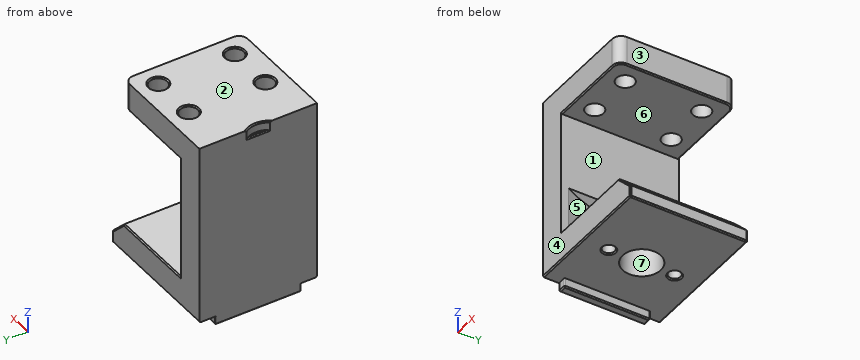
from build123d import *

# Parameters (mm, degrees)
SKETCH_1_R          = 3.2375
EXTRUDE_1_DEPTH     = 5
SKETCH_2_R          = 1.015
CUT_EXTRUDE_1_DEPTH = 2.85
CHAMFER_1_SIZE      = 0.2
EXTRUDE_2_DEPTH     = 1.55
CHAMFER_2_SIZE      = 0.2
FILLET_1_R          = 0.15
SKETCH_6_W          = 4.8
SKETCH_6_H          = 20
EXTRUDE_3_DEPTH     = 31
EXTRUDE_START       = 31
SKETCH_7_W          = 19.9
SKETCH_7_H          = 20
EXTRUDE_4_DEPTH     = 4.92
CUT_EXTRUDE_START   = 26.08
SKETCH_8_R          = 1.52
CUT_EXTRUDE_2_DEPTH = 4.92
CHAMFER_3_SIZE      = 0.2
CUT_EXTRUDE_START_2 = 31
CUT_EXTRUDE_3_DEPTH = 31
FILLET_2_R          = 1.5
CUT_EXTRUDE_4_DEPTH = 1.5
CHAMFER_4_SIZE      = 0.2
SKETCH_13_W         = 3.2
SKETCH_13_H         = 20
EXTRUDE_5_DEPTH     = 5
CHAMFER_5_SIZE      = 3
CUT_EXTRUDE_START_3 = 5
CUT_EXTRUDE_5_DEPTH = 7
CHAMFER_7_SIZE      = 1.3
CHAMFER_8_SIZE      = 0.2


with BuildPart() as part:
    # 草图1 → 凸台-拉伸1 (new body)
    with BuildSketch(Plane.XY):
        Polygon((13.5775, 0), (13.5775, 10), (-10.48, 10), (-10.48, 0), (-10.48, -10), (13.5775, -10), align=None)
        Circle(SKETCH_1_R, mode=Mode.SUBTRACT)
    extrude(amount=EXTRUDE_1_DEPTH)

    # 草图2 → 切除-拉伸1 (cut)
    with BuildSketch(Plane.XY):
        with Locations((0, 5.6)):
            Circle(SKETCH_2_R)
        with Locations((0, -5.6)):
            Circle(SKETCH_2_R)
    extrude(amount=CUT_EXTRUDE_1_DEPTH, mode=Mode.SUBTRACT)

    # 倒角1
    chamfer_1_edges = [part.edges().sort_by_distance(p)[0] for p in [
        (-1.015, 5.6, 0),
        (-1.015, -5.6, 0),
    ]]
    chamfer(chamfer_1_edges, length=CHAMFER_1_SIZE)

    # 草图5 → 凸台-拉伸2 (add)
    with BuildSketch(Plane.XY):
        Polygon((-9, 7.275), (-10.48, 7.275), (-10.48, -7.275), (-9, -7.275), (-9, 0), align=None)
    extrude(amount=-EXTRUDE_2_DEPTH)

    # 倒角2
    chamfer_2_edges = [part.edges().sort_by_distance(p)[0] for p in [
        (-9.74, -7.275, -1.55),
        (-10.48, 0, -1.55),
        (-9.74, 7.275, -1.55),
        (-9, 0, -1.55),
    ]]
    chamfer(chamfer_2_edges, length=CHAMFER_2_SIZE)

    # 圆角1
    fillet_1_edges = [part.edges().sort_by_distance(p)[0] for p in [
        (-10.48, -7.275, -0.675),
        (-9, -7.275, -0.675),
        (-9, 7.275, -0.675),
        (-10.48, 7.275, -0.675),
    ]]
    fillet(fillet_1_edges, radius=FILLET_1_R)

    # 草图6 → 凸台-拉伸3 (add)
    with BuildSketch(Plane.XY):
        with Locations((-8.08, 0)):
            Rectangle(SKETCH_6_W, SKETCH_6_H)
    extrude(amount=EXTRUDE_3_DEPTH)

    # 草图7 → 凸台-拉伸4 (add)
    with BuildSketch(Plane.XY.offset(EXTRUDE_START)):
        with Locations((3.6275, 0)):
            Rectangle(SKETCH_7_W, SKETCH_7_H)
    extrude(amount=-EXTRUDE_4_DEPTH)

    # 草图8 → 切除-拉伸2 (cut)
    with BuildSketch(Plane.XY.offset(CUT_EXTRUDE_START)):
        with Locations((-2.3025, 6.5)):
            Circle(SKETCH_8_R)
        with Locations((5.6975, 6.5)):
            Circle(SKETCH_8_R)
        with Locations((5.6975, -6.5)):
            Circle(SKETCH_8_R)
        with Locations((-2.3025, -6.5)):
            Circle(SKETCH_8_R)
    extrude(amount=CUT_EXTRUDE_2_DEPTH, mode=Mode.SUBTRACT)

    # 倒角3
    chamfer_3_edges = [part.edges().sort_by_distance(p)[0] for p in [
        (-3.8225, -6.5, 31),
        (4.1775, -6.5, 31),
        (4.1775, 6.5, 31),
        (-3.8225, 6.5, 31),
    ]]
    chamfer(chamfer_3_edges, length=CHAMFER_3_SIZE)

    # 草图10 → 切除-拉伸3 (cut)
    with BuildSketch(Plane.XY.offset(CUT_EXTRUDE_START_2)):
        Polygon((9.198987738, 6.5), (9.198987738, -10), (13.5775, -10), (13.5775, 10), (9.198987738, 10), align=None)
    extrude(amount=-CUT_EXTRUDE_3_DEPTH, mode=Mode.SUBTRACT)

    # 圆角2
    fillet_2_edges = [part.edges().sort_by_distance(p)[0] for p in [
        (9.198987738, 10, 28.54),
        (9.198987738, -10, 28.54),
    ]]
    fillet(fillet_2_edges, radius=FILLET_2_R)

    # 草图11 → 切除-拉伸4 (cut)
    with BuildSketch(Plane.XY.offset(CUT_EXTRUDE_START_2)):
        with BuildLine():
            Line((-10.48, 2.007504789), (-10.48, -2.007504789))
            ThreePointArc((-10.48, -2.007504789), (-9.862877127, 0), (-10.48, 2.007504789))
        make_face()
    extrude(amount=-CUT_EXTRUDE_4_DEPTH, mode=Mode.SUBTRACT)

    # 倒角4
    chamfer_4_edges = [part.edges().sort_by_distance(p)[0] for p in [
        (1.009493869, 10, 26.08),
        (1.009493869, -10, 26.08),
        (9.198987738, 0, 26.08),
        (8.759647909, 9.560660172, 26.08),
        (8.759647909, -9.560660172, 26.08),
        (-10.48, 0, 29.5),
        (-9.862877127, 0, 31),
    ]]
    chamfer(chamfer_4_edges, length=CHAMFER_4_SIZE)

    # 草图13 → 凸台-拉伸5 (add)
    with BuildSketch(Plane.XY):
        with Locations((10.798987738, 0)):
            Rectangle(SKETCH_13_W, SKETCH_13_H)
    extrude(amount=EXTRUDE_5_DEPTH)

    # 倒角5
    chamfer_5_edges = [part.edges().sort_by_distance(p)[0] for p in [
        (12.398987738, 0, 5),
    ]]
    chamfer(chamfer_5_edges, length=CHAMFER_5_SIZE)

    # 草图14 → 切除-拉伸5 (cut)
    with BuildSketch(Plane.XY.offset(CUT_EXTRUDE_START_3)):
        with BuildLine():
            Line((-5.284271247, 10), (-5.284271247, -10))
            ThreePointArc((-5.284271247, -10), (-7, 0), (-5.284271247, 10))
        make_face()
    extrude(amount=CUT_EXTRUDE_5_DEPTH, mode=Mode.SUBTRACT)

    # 倒角7
    chamfer_7_edges = [part.edges().sort_by_distance(p)[0] for p in [
        (-5.68, 0, 12),
    ]]
    chamfer(chamfer_7_edges, length=CHAMFER_7_SIZE)

    # 倒角8
    chamfer_8_edges = [part.edges().sort_by_distance(p)[0] for p in [
        (1.859493869, -10, 5),
        (0.959493869, 10, 0),
        (12.398987738, 0, 0),
        (12.398987738, 10, 1),
        (12.398987738, -10, 1),
        (10.898987738, -10, 3.5),
        (1.859493869, 10, 5),
        (10.898987738, 10, 3.5),
        (0.959493869, -10, 0),
    ]]
    chamfer(chamfer_8_edges, length=CHAMFER_8_SIZE)


solid = part.part
Input: part model. Units: mm. Frame: model coordinates. Face numbers are marked on the shaded views. A direction names the side the tool comes from. Coordinates: 2 decimals unless noted, no trailing zeros. Loops run counter-clockwise (first coordinate to the right, second up) from the corner with the lowest first, then second, coordinate; pieces in that order, holes last.
Q1. Cut plane D-D (y = -6). Give the number of separate pieces and of enclosed holes in the cut face, then the cut area to 3 significant figures.
Q2. Set-up query: the marked faces 4, 5, 6 and 7. Return all of +Z, -Z, +X, -X, +Y, -Y with unobstructed straight access to the full face (end or side cutting, diameter ignored); none if empty.
Q3. Draft query along Z for the marked faces 1, 2 and 3. Return one class per face: +Z half, -Z half, draft (parallel to the pull), parting line (faces both ways), or undercut.
Q4. Contact query for flat-ended pins moving along their axis: pin 1 (11.5 mm diameter, centred on x = 1.5, y = -4, fed in from -Z); pin 2 (1.5 mm diameter, centred on x = 9.5, y = -4.5, fed in from +Z); pin 3 (1.4 mm diameter, centred on y = -3.5, z = 29, fed in from +X); pin 4 (6 mm diameter, centred on y = 0.5, z = 22, fed in from +X). Output: stop coordinate, or through.
Q5. Cut plane C-C (x = 11). Output: boundary loops of the cut face in (y, z), then the cut area to 3 significant figures.
Q6. Cut plane B-B (z = 5.5). Output: boundary loops of the cut face in (x, y).
Q7. Material intervals for line 1 (Y direction, x = 0, z = 1.4) (1 decimal); line 2 (Z direction, x = 7.5, y = 2.75); line 3 (Z direction, x = -0.75, y = 5.5), sorted ascending.
Working result:
1. separate pieces: 3
1. enclosed holes: 0
1. area: 271 mm2
2. face 4: +Z, -Z, +X, -X, -Y
2. face 5: +X
2. face 6: +X, +Y, -Y
2. face 7: -Z
3. face 1: undercut
3. face 2: +Z half
3. face 3: draft
4. pin 1: stops at z = 0
4. pin 2: stops at z = 31
4. pin 3: stops at x = 9.2
4. pin 4: stops at x = -5.68
5. outline: (-10, 0.2) - (-9.8, 0) - (9.8, 0) - (10, 0.2) - (10, 3.12) - (9.8, 3.4) - (-9.8, 3.4) - (-10, 3.12) - close
5. area: 67.9 mm2
6. outline: (-10.48, -10) - (-5.68, -10) - (-5.68, -8.8) arc R30 cw to (-5.68, 8.8) - (-5.68, 10) - (-10.48, 10) - close
7. line 1: y = -10 to -6.6, -4.6 to -3.2, 3.2 to 4.6, 6.6 to 10
7. line 2: z = 0 to 5, 26.08 to 31
7. line 3: z = 2.85 to 5, 26.08 to 31
